Source: three-view drawing plus pictorial views. Frame: mm from the lowest corner of the part. Give positions to 0.01 mm unless a question says otherwise; leave off trailing zeros. Write each loop counter-clockwise with the first axis right and the second up, starting at its lowest first coordinate (ties: lowest second). Pieces come first, ordered by that corner, then holes.
Q1. Cut plane C-C on x = 9. Return the cut outline in (y, z), plus the area to 3 significant figures.
Q2. Cut plane A-A on y = 20.75. Return the cut outline in (x, z).
Q3. Line query: L1, parallel to X at y = 5.5, z = 2.9; L2, parallel to Y at x = 24.5, z = 0.3; L3, parallel to X at y = 12.75, z = 1.1. Output: solid intervals per line, ascending.
Q4. Cut plane D-D on y = 23.5. Return the cut outline in (x, z), plus the area to 3 significant figures.
Q5. Cut plane B-B on z = 1.5. Return the cut outline in (x, y).
Q6. Pin query (flat end, axial travel): pin 1 (0.9 mm diameter, centred on x = 32.5, z = 2, fed in from -Y); pin 2 (1.5 mm diameter, centred on y = 14.5, z = 1.5, fed in from -X); pin 3 (0.9 mm diameter, centred on x = 28.5, z = 1.5, fed in from +Y). Return the tip coordinate at first contact, or that it passes through.
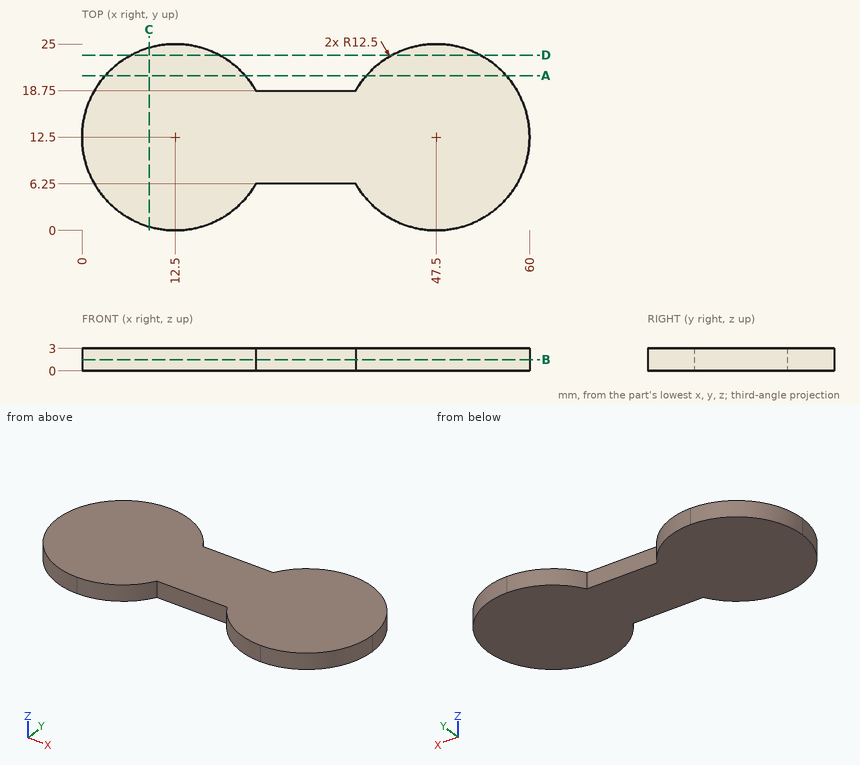
Data:
1. outline: (0.5, 0) - (24.5, 0) - (24.5, 3) - (0.5, 3) - close
1. area: 72.0 mm2
2. outline: (3.11, 0) - (21.89, 0) - (21.89, 3) - (3.11, 3) - close; (38.11, 0) - (56.89, 0) - (56.89, 3) - (38.11, 3) - close
3. L1: x = 2.14 to 22.86, 37.14 to 57.86
3. L2: y = 6.25 to 18.75
3. L3: x = 0 to 60
4. outline: (6.56, 0) - (18.44, 0) - (18.44, 3) - (6.56, 3) - close; (41.56, 0) - (53.44, 0) - (53.44, 3) - (41.56, 3) - close
4. area: 71.2 mm2
5. outline: (23.33, 6.25) - (36.67, 6.25) arc R12.5 ccw (long way) to (36.67, 18.75) - (23.33, 18.75) arc R12.5 ccw (long way) to start
6. pin 1: stops at y = 6.25
6. pin 2: stops at x = 0.06
6. pin 3: stops at y = 18.75
